Input: dimensioned drawing with shaded views. Units: mm. Origin: part minimum x, y, z. A direction names the side the tool comes from. Give positions to 0.01 mm unless a question says otherwise; leave off trailing zeros. Write each loop counter-clockwise with the first axis right and the second up, starting at its lowest first coordinate (ties: lowest second). Pieces come first, ordered by that corner, then holes.
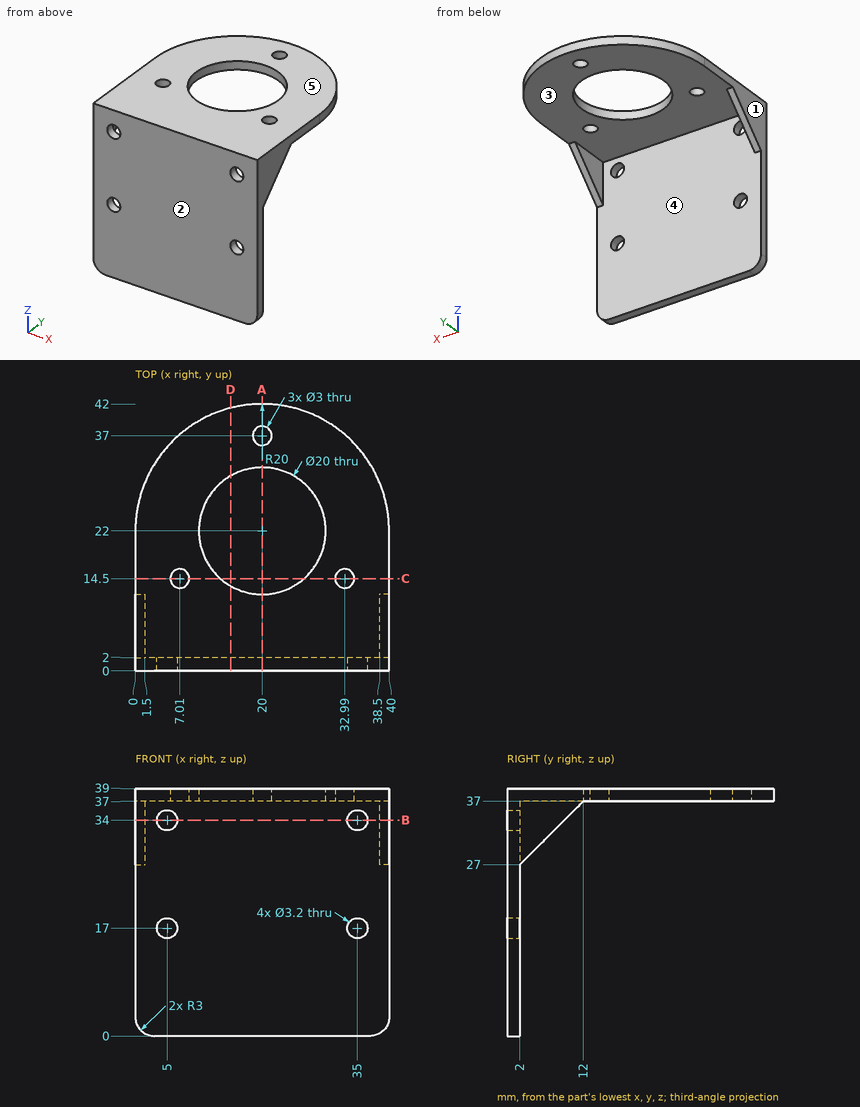
Item 1: Section B-B (z = 34). Return loops of the section in (x, y).
Item 2: Section C-C (y = 14.5). Return loops of the section in (x, z) (1 decimal).
Item 3: Section A-A (x = 20). Return loops of the section in (y, z).
Item 4: Ray query, line 1 (Z direction, x = 35, y = 0.9); line 2 (X direction, y = 4, z = 34); line 3 (Z direction, x = 35, y = 29). Return the intervals inside material, ascending.
Item 5: Set-up query: the marked faces 4 and 5. Return all of +Z, -Z, +X, -X, +Y, -Y with unobstructed straight access to the full face (end or side cutting, diameter ignored); none if empty.
Item 6: Mould query, pull axis X, two halves, no side actions, for the marked faces 1, 2 and 3. Classes: +X half, -X half, draft (parallel to the pull), parting line (faces both ways), or undercut.
Item 7: Pin query (flat end, axial travel): pin 1 (1 mm diameter, centred on x = 11, z = 18, fed in from +Y); pin 2 (3.5 mm diameter, centred on x = 20, y = 37, fed in from -Z); pin 3 (2.5 mm diameter, centred on x = 35, z = 34, fed in from -Y). Return the tip coordinate at first contact, or that it passes through.
Item 8: Section D-D (x = 15). Return loops of the section in (y, z) (1 decimal), and give its area (3 significant figures).
Solved:
1. outline: (0, 0) - (3.4, 0) - (3.4, 2) - (1.5, 2) - (1.5, 9) - (0, 9) - close; (6.6, 0) - (33.4, 0) - (33.4, 2) - (6.6, 2) - close; (36.6, 0) - (40, 0) - (40, 9) - (38.5, 9) - (38.5, 2) - (36.6, 2) - close
2. outline: (0, 37) - (5.5, 37) - (5.5, 39) - (0, 39) - close; (8.5, 37) - (13.4, 37) - (13.4, 39) - (8.5, 39) - close; (26.6, 37) - (31.5, 37) - (31.5, 39) - (26.6, 39) - close; (34.5, 37) - (40, 37) - (40, 39) - (34.5, 39) - close
3. outline: (0, 0) - (2, 0) - (2, 37) - (12, 37) - (12, 39) - (0, 39) - close; (32, 37) - (35.5, 37) - (35.5, 39) - (32, 39) - close; (38.5, 37) - (42, 37) - (42, 39) - (38.5, 39) - close
4. line 1: z = 0 to 15.4, 18.6 to 32.4, 35.6 to 39
4. line 2: x = 0 to 1.5, 38.5 to 40
4. line 3: z = 37 to 39
5. face 4: -Z, +Y
5. face 5: +Z, +X, -X, +Y, -Y
6. face 1: -X half
6. face 2: draft
6. face 3: undercut
7. pin 1: stops at y = 2
7. pin 2: stops at z = 37
7. pin 3: passes through
8. outline: (0, 0) - (2, 0) - (2, 37) - (13.3, 37) - (13.3, 39) - (0, 39) - close; (30.7, 37) - (41.4, 37) - (41.4, 39) - (30.7, 39) - close
8. area: 122 mm2
